Read the model definition and answer for the solid it produces. Units are mm, in the model's axes. A direction names the side the tool comes from. Round coordinates to 2 decimals unless told otherwise and drop trailing zeros. Write each loop counter-clockwise with the first axis right and the second up, starting at its lowest first coordinate (ties: lowest second). Pieces come first, ordered by that corner, then holes.
from build123d import *

# Parameters (mm, degrees)
BOSS_EXTRUDE1_DEPTH = 12.7
FILLET1_R           = 2.54


with BuildPart() as part:
    # Sketch1 → Boss-Extrude1 (new body)
    with BuildSketch(Plane.XY):
        Polygon((0, 0), (0, -4.191), (-1.55575, -4.191), (-1.55575, -7.112), (0, -7.112), (0, -10.287), (10.6045, -10.287), (10.6045, -7.112), (12.16025, -7.112), (12.16025, -4.191), (10.6045, -4.191), (10.6045, 0), (18.97725, 0), (18.97725, 19.558), (15.80225, 19.558), (15.80225, 3.089), (-6.858, 3.089), (-6.858, 0), align=None)
    extrude(amount=BOSS_EXTRUDE1_DEPTH)

    # Fillet1
    fillet1_edges = [part.edges().sort_by_distance(p)[0] for p in [
        (15.80225, 3.089, 6.35),
    ]]
    fillet(fillet1_edges, radius=FILLET1_R)


solid = part.part
Q1. Flat-ended cylindrical pins translate along their axes: pin 1 Ø1.3 at (y, z) = (-2.5, 5.5) entering from +X; pin 2 Ø3.5 at (y, z) = (-3, 7.5) entering from -X; pin 3 Ø3.5 at (x, z) = (-4, 5.5) entering from -Y. Find the tip coordinate at first contact, or state that the pin passes through.
Verdict:
pin 1: stops at x = 10.6
pin 2: stops at x = -1.56
pin 3: stops at y = 0
Q2. Which of the six approach directions +Z, -Z, +X, -X, +Y, -Y give full straight-line access (tool end or side, diameter ignored) to faces 1 (the flat face through (10.604, -9, 6)), 2 (the flat face through (-3, 0, 6)), 3 (the flat face through (15.802, 13, 6)), 4 (the flat face through (-1.556, -6, 6)), 5 (the flat face through (15, 0, 6))?
Verdict:
face 1: +Z, -Z, +X, -Y
face 2: +Z, -Z, -X
face 3: +Z, -Z, -X, +Y
face 4: +Z, -Z, -X, -Y
face 5: +Z, -Z, +X
Q3. Section B-B (z = 8.5) is taken. Determine the outline of the cut face in (x, y), then the cut area to 3 significant figures.
Verdict:
outline: (-6.86, 0) - (0, 0) - (0, -4.19) - (-1.56, -4.19) - (-1.56, -7.11) - (0, -7.11) - (0, -10.29) - (10.6, -10.29) - (10.6, -7.11) - (12.16, -7.11) - (12.16, -4.19) - (10.6, -4.19) - (10.6, 0) - (18.98, 0) - (18.98, 19.56) - (15.8, 19.56) - (15.8, 5.63) arc R2.54 cw to (13.26, 3.09) - (-6.86, 3.09) - close
area: 252 mm2
Q4. Section A-A (x = 11) is taken. Determine the outline of the cut face in (y, z), then the cut area to 3 significant figures.
Verdict:
outline: (-7.11, 0) - (-4.19, 0) - (-4.19, 12.7) - (-7.11, 12.7) - close; (0, 0) - (3.09, 0) - (3.09, 12.7) - (0, 12.7) - close
area: 76.3 mm2
Q5. Section D-D (y = 10.5) is taken. Determine the outline of the cut face in (x, z).
Verdict:
outline: (15.8, 0) - (18.98, 0) - (18.98, 12.7) - (15.8, 12.7) - close
Q6. Determine the mould class of faces 6 (the flat face through (3, 3.089, 6)), 7 (the flat face through (-1, -4.191, 6)), 8 (the flat face through (7, 0, 0)) for opening direction Y: pulls with the +Y half, pulls with the -Y half, needs draft (parallel to the pull), parting line crosses it, or undercut.
Verdict:
face 6: pulls with the +Y half
face 7: undercut
face 8: needs draft
Q7. Section C-C (x = -2) is taken. Determine the outline of the cut face in (y, z).
Verdict:
outline: (0, 0) - (3.09, 0) - (3.09, 12.7) - (0, 12.7) - close
Q8. Straight lines are drawn through the part: probe 1 along Y at (x, z) = (7, 1); probe 2 along X at (y, z) = (10, 10.5); probe 3 along Y at (x, z) = (12.75, 8). For each, find the intervals that lie inside material, in ascending order.
Verdict:
probe 1: y = -10.29 to 3.09
probe 2: x = 15.8 to 18.98
probe 3: y = 0 to 3.09
